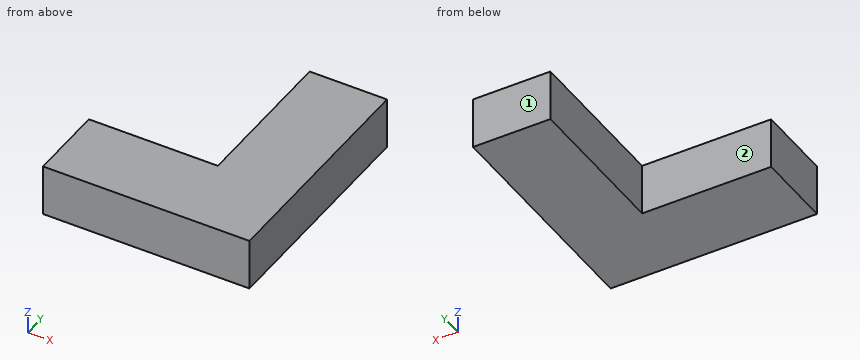
Autodesk Fusion 360 part; units mm, degrees
sketch "Sketch1" plane through (0, 0, 0) normal (0, 0, 1) x (1, 0, 0)
  line L0 (0, 0) -> (35, 0)
  line L1 (35, 0) -> (35, 15)
  line L2 (35, 15) -> (0, 15)
  line L3 (0, 15) -> (0, 0)
  line L4 (25, 0) -> (40, 0)
  line L5 (40, 0) -> (40, 45)
  line L6 (40, 45) -> (25, 45)
  line L7 (25, 45) -> (25, 0)
extrude "Extrude1" add sketch "Sketch1" along normal blind 10
sketch "Sketch2" plane through (0, 0, 0) normal (0, 1, 0) x (1, 0, 0)
Design review of the part built by this model. Coordinates are the model's own, in mm. Face numbers are marked on the shaded views. A direction names the side the tool comes from. Round coordinates to 2 decimals unless told otherwise and drop trailing zeros. Write each loop counter-clockwise with the first axis right and the second up, starting at its lowest first coordinate (ties: lowest second). Pieces come first, ordered by that corner, then holes. Notation, with made-up numbers: (-34, 58.25) -> (23, 58.25) arc R19 ccw to (23, 65.25) -> close; hole circle Ø8 at (-32, 55). An arc over 180 degrees is marked (long way). One line per question, with ' | ' between items.
(1) Insertion check: P1, Ø10, axis at x = 10.5, y = 22.5, coming from the -Z side; P2, Ø5, axis at x = 14.5, z = 7.5, coming from the +Y side; P3, Ø1.5, axis at y = 19.5, z = 7, coming from the -X side. Each pin has a flat end and moves straight along its axis. Give the tip position at first contact, or say it passes through.
Result sheet:
P1: through | P2: y = 15 | P3: x = 25
(2) Take a section at B-B, the plane y = 21. State the section outline as (x, z) points, and give its area (3 significant figures).
Result sheet:
outline: (25, 0) -> (40, 0) -> (40, 10) -> (25, 10) -> close | area: 150 mm2
(3) Take a section at A-A, the plane z = 1.5. State the section outline as (x, y) points, and give its area (3 significant figures).
Result sheet:
outline: (0, 0) -> (40, 0) -> (40, 45) -> (25, 45) -> (25, 15) -> (0, 15) -> close | area: 1,050 mm2
(4) Take a section at C-C, the plane x = 15.5. State the section outline as (y, z) points, and give its area (3 significant figures).
Result sheet:
outline: (0, 0) -> (15, 0) -> (15, 10) -> (0, 10) -> close | area: 150 mm2
(5) Wall thickness on line 1 (X direction, y = 21, z = 5); line 2 (Y direction, x = 18.5, z = 0.5): over which ranges is each line inside the solid? List them lowest first. Write a range as [from, to].
Result sheet:
line 1: [25, 40] | line 2: [0, 15]
(6) Machinability: for the marked faces 1 and 2, which of the approach directions +Z, -Z, +X, -X, +Y, -Y give a long, thin tool a straight path to every point of the face, cutting with its end or side? Answer none if there is none.
Result sheet:
face 1: +Z, -Z, +X, -X, +Y | face 2: +Z, -Z, -X, +Y
